from build123d import *

# Parameters (mm, degrees)
SKETCH1_W           = 19.05
SKETCH1_H           = 19.05
SKETCH1_R           = 4.7625
BOSS_EXTRUDE1_DEPTH = 3.175


with BuildPart() as part:
    # Sketch1 → Boss-Extrude1 (new body)
    with BuildSketch(Plane(origin=(0, 0, 0), x_dir=(0, 0, -1), z_dir=(1, 0, 0))):
        Rectangle(SKETCH1_W, SKETCH1_H)
        Circle(SKETCH1_R, mode=Mode.SUBTRACT)
    extrude(amount=BOSS_EXTRUDE1_DEPTH)


solid = part.part
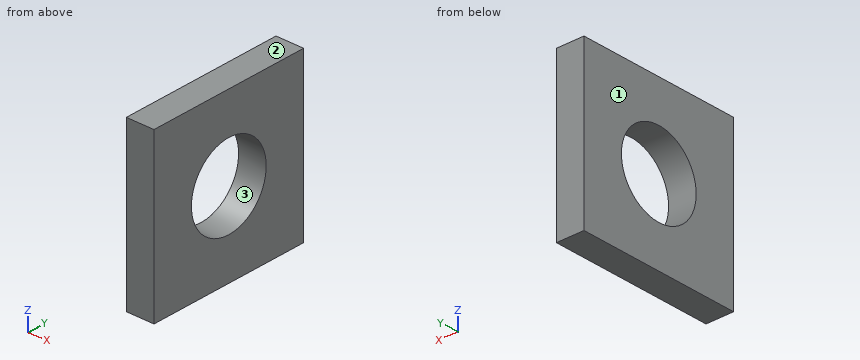
The model under review builds one solid part; all positions refer to its coordinate system, in mm. Face numbers are marked on the shaded views. Round coordinates to 2 decimals unless told otherwise and drop trailing zeros. Write each loop counter-clockwise with the first axis right and the second up, starting at its lowest first coordinate (ties: lowest second). Pieces come first, ordered by that corner, then holes. Notation, with made-up numbers: M -13,63 L 26,63 A4 cw 26,68 Z; hole C 77,59 d2. An arc over 180 degrees is marked long. Use a Markdown table: item, result. Add a question column.
Q1. We need section A-A, the plane y = 0. State the section outline as (x, z) points (1 decimal), plus the area to 3 significant figures.
Q2. To check wall thickness, follow line 1 (Y direction, x = 1.85, z = 0) (1 decimal); line 2 (Y direction, x = 0.2, z = -1) (3 decimals); line 3 (Z direction, x = 0.3, y = 0.75) (3 decimals). State the ranges of each line that lie inside material, in increasing order.
Q3. Insertion check: pin 1 (1 mm diameter, centred on y = -3, z = -1, fed in from -X). The pin has a flat end and moves straight along its axis. Give the tip position at first contact, or say it passes through.
Q4. The part is to be moulded in two halves that separate along Z. For the marked faces 1, 2 and 3, say which applies: pulls with the +Z half, pulls with the -Z half, needs draft (parallel to the pull), parting line crosses it, or undercut.
Q5. We need section C-C, the plane x = 2.4. State the section outline as (y, z) points (1 decimal).
Findings below:
| question | item | result |
|---|---|---|
| 1 | outline | M 0,-9.5 L 3.2,-9.5 L 3.2,-4.8 L 0,-4.8 Z; M 0,4.8 L 3.2,4.8 L 3.2,9.5 L 0,9.5 Z |
| 1 | area | 30.2 mm² |
| 2 | line 1 | y = -9.5 to -4.8, 4.8 to 9.5 |
| 2 | line 2 | y = -9.525 to -4.656, 4.656 to 9.525 |
| 2 | line 3 | z = -9.525 to -4.703, 4.703 to 9.525 |
| 3 | pin 1 | passes through |
| 4 | face 1 | needs draft |
| 4 | face 2 | pulls with the +Z half |
| 4 | face 3 | undercut |
| 5 | outline | M -9.5,-9.5 L 9.5,-9.5 L 9.5,9.5 L -9.5,9.5 Z; hole C 0,0 d9.5 |
